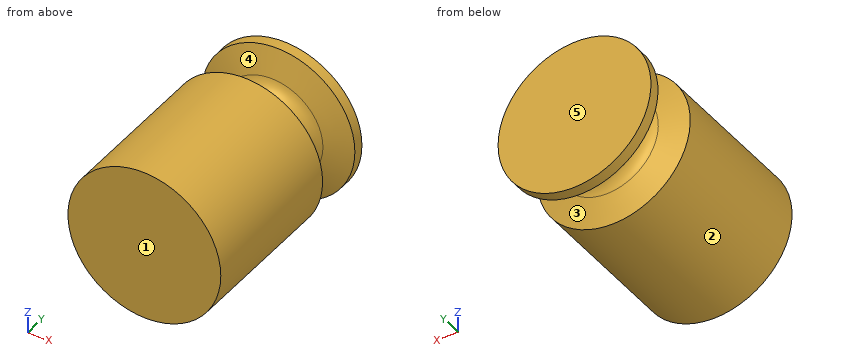
```python
from build123d import *

# Parameters (mm, degrees)
SKETCH1_R           = 25
BOSS_EXTRUDE1_DEPTH = 70


with BuildPart() as part:
    # Sketch1 → Boss-Extrude1 (new body)
    with BuildSketch(Plane(origin=(0, 0, 0), x_dir=(1, 0, 0), z_dir=(0, 1, 0))):
        Circle(SKETCH1_R)
    extrude(amount=BOSS_EXTRUDE1_DEPTH)

    # Sketch2 → Cut-Revolve1 (revolve, cut)
    with BuildSketch(Plane(origin=(0, 0, 0), x_dir=(0, 0, -1), z_dir=(1, 0, 0))):
        with BuildLine():
            Line((25, 50.5), (16.532991719, 53.5))
            ThreePointArc((16.532991719, 53.5), (13.972369333, 55.438871512), (13, 58.5))
            ThreePointArc((13, 58.5), (13.972369333, 61.561128488), (16.532991719, 63.5))
            Line((16.532991719, 63.5), (25, 66.5))
            Line((25, 66.5), (25, 50.5))
        make_face()
    revolve(axis=Axis((0, 73.5, 0), (0, -1, 0)), mode=Mode.SUBTRACT)


solid = part.part
```
Verification items for the finished model (mm, model axes). Face numbers are marked on the shaded views. A direction names the side the tool comes from. Give positions to 0.01 mm unless a question says otherwise; leave off trailing zeros. Loops run counter-clockwise (first coordinate to the right, second up) from the corner with the lowest first, then second, coordinate; pieces in that order, holes last. Notation, with made-up numbers: M 58,89 L 116,89 A13 cw 116,98 Z; hole C 55,72 d2. An arc over 180 degrees is marked long. One line per question, with ' | ' between items.
Item 1: Thickness scan on line 1 (Y direction, x = 13, z = 12.5); line 2 (Y direction, x = 20, z = 8); line 3 (Z direction, x = 0, y = 33.5). Record the ranges inside material, lowest first. Write a range as [from, to].
Completed:
line 1: y = [0, 52.97], [64.03, 70] | line 2: y = [0, 51.73], [65.27, 70] | line 3: z = [-25, 25]
Item 2: Section check A-A, the plane y = 44. Record the cut outline in (x, z).
Completed:
outline: C 0,0 d50
Item 3: Draft check along Y on the marked faces 1, 2 and 3. Enter one of: +Y half, -Y half, draft (parallel to the pull), parting line (faces both ways), or undercut.
Completed:
face 1: -Y half | face 2: draft | face 3: undercut
Item 4: Tool access check on the marked faces 4 and 5. Record the directions out of +Z, -Z, +X, -X, +Y, -Y that give a thin tool (end or side, any length) a straight path to the whole face; none if there is none.
Completed:
face 4: none | face 5: +Z, -Z, +X, -X, +Y
Item 5: Depth check by flat-ended pin: P1, Ø2, axis at x = 6, y = 46.5, coming from the +Z side; P2, Ø2, axis at x = -7.5, y = 31.5, coming from the +Z side; P3, Ø1, axis at x = -17.5, y = 31.5, coming from the -Z side. Enter the tip coordinate at first touch or a pass-through.
Completed:
P1: stops at z = 24.49 | P2: stops at z = 24.14 | P3: stops at z = -18.33
